Can you work these out from the model? Positions are in its coordinate system, mm. A direction names the side the tool comes from. Round coordinates to 2 decimals unless told otherwise and drop trailing zeros. Order: outer loops, then holes, each group sorted by start corner. A loop starts at its lowest first (then second) coordinate and runs counter-clockwise, first axis right, second up. Notation, with made-up numbers: (-32.5, 7.25) -> (-15.5, 7.25) arc R18 cw to (-15.5, 26.25) -> close; hole circle Ø1 at (14.25, 44.5). An arc over 180 degrees is marked (long way). One line per item, written item: value.
```python
from build123d import *

# Parameters (mm, degrees)
BOSS_EXTRUDE1_DEPTH = 3
SKETCH3_R           = 5.025
CUT_EXTRUDE1_DEPTH  = 71.697893831


with BuildPart() as part:
    # Sketch1 → Boss-Extrude1 (new, symmetric)
    with BuildSketch(Plane(origin=(0, 0, 0), x_dir=(0, 0, -1), z_dir=(1, 0, 0))):
        with BuildLine():
            Line((0, 66), (-15, 66))
            Line((-15, 66), (-15, 62.56))
            ThreePointArc((-15, 62.56), (-17.468868001, 47.38033448), (-24.620970576, 33.765453531))
            ThreePointArc((-24.620970576, 33.765453531), (-13.706982887, 8.251900539), (-16, -19.403091525))
            Line((-16, -19.403091525), (-13.500700251, -20.50145429))
            Line((-13.500700251, -20.50145429), (-16, -24.97))
            Line((-16, -24.97), (-16, -66))
            Line((-16, -66), (0, -66))
            Line((0, -66), (0, 66))
        make_face()
    extrude(amount=BOSS_EXTRUDE1_DEPTH, both=True)

    # Sketch3 → Cut-Extrude1 (cut, through all)
    with BuildSketch(Plane(origin=(3, 0, 0), x_dir=(0, 0, -1), z_dir=(1, 0, 0))):
        with Locations((-8, 51)):
            Circle(SKETCH3_R)
        with Locations((-8, -54)):
            Circle(SKETCH3_R)
    extrude(amount=-CUT_EXTRUDE1_DEPTH, mode=Mode.SUBTRACT)


solid = part.part
```
Q1. We'd pull the mould along Y, two halves only. Please class faces 1 (the face through (0, -66, 8)), 2 (the face through (0.042, -58.458, 5.681)), 3 (the face through (0, -1, 0)): released by +Y, released by -Y, zero draft, split by the parting line, or undercut.
Answers below:
face 1: released by -Y
face 2: undercut
face 3: zero draft
Q2. I want a section at B-B on z = 8. List the corners of the cut face in (x, y) for me (3 decimals).
Answers below:
outline: (-3, -66) -> (3, -66) -> (3, -59.025) -> (-3, -59.025) -> close; (-3, -48.975) -> (3, -48.975) -> (3, 45.975) -> (-3, 45.975) -> close; (-3, 56.025) -> (3, 56.025) -> (3, 66) -> (-3, 66) -> close
Q3. On a 3-axis mill with a long thin cutter (end or side, diameter ignored), from which of +Z, -Z, +X, -X, +Y, -Y can I reach the whole of each face in a straight line? I mean faces 4 (the face through (0, 64, 15)), 5 (the face through (0.042, -19.945, 14.768)), 6 (the face through (0, -45, 16)). Say none if no direction works.
Answers below:
face 4: +Z, +X, -X, +Y
face 5: +Z, +X, -X
face 6: +Z, +X, -X, -Y
Q4. I want a section at D-D on y = 51. List the corners of the cut face in (x, z) for me (3 decimals), plus the area to 3 significant figures.
Answers below:
outline: (-3, 0) -> (3, 0) -> (3, 2.975) -> (-3, 2.975) -> close; (-3, 13.025) -> (3, 13.025) -> (3, 16.416) -> (-3, 16.416) -> close
area: 38.2 mm^2
Q5. Will these pins go through, and if not, where does the flat tip stop? pin 1 Ø3 at (x, y) = (-1, 44) entering from +Z; pin 2 Ø3 at (x, y) = (0.5, -40) entering from +Z.
Answers below:
pin 1: z = 19.4
pin 2: z = 16
Q6. I want a section at C-C on x = -1.4. List the corners of the cut face in (y, z) for me (3 decimals).
Answers below:
outline: (-66, 0) -> (66, 0) -> (66, 15) -> (62.56, 15) arc R47.9 cw to (33.765, 24.621) arc R57.555 cw to (-19.403, 16) -> (-20.501, 13.501) -> (-24.97, 16) -> (-66, 16) -> close; hole circle Ø10.05 at (-54, 8); hole circle Ø10.05 at (51, 8)
Q7. I want a section at A-A on y = -54. List the corners of the cut face in (x, z) for me (3 decimals), plus the area to 3 significant figures.
Answers below:
outline: (-3, 0) -> (3, 0) -> (3, 2.975) -> (-3, 2.975) -> close; (-3, 13.025) -> (3, 13.025) -> (3, 16) -> (-3, 16) -> close
area: 35.7 mm^2
Q8. Please list where these lines run through material, in increasing order: line 1 along Y through (x, z) = (0.55, 8) (3 decimals); line 2 along Y through (x, z) = (1.9, 6.5); line 3 along Z through (x, y) = (-2.1, -47).
Answers below:
line 1: -66 to -59.025, -48.975 to 45.975, 56.025 to 66
line 2: -66 to -58.8, -49.2 to 46.2, 55.8 to 66
line 3: 0 to 16
